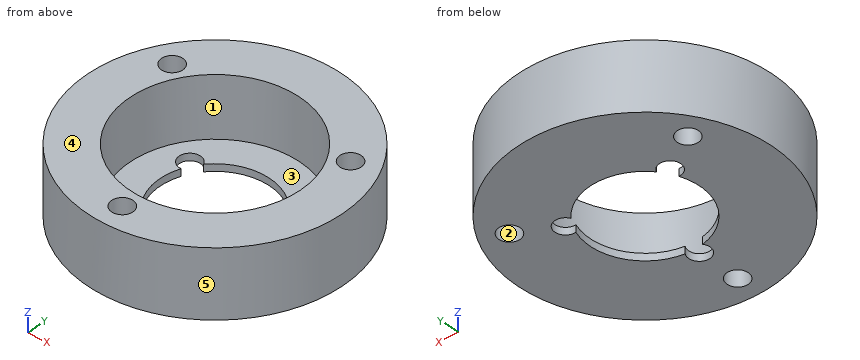
```python
from build123d import *

# Parameters (mm, degrees)
ESQUISSE1_W      = 50
ESQUISSE1_H      = 9.5
EXTRUSION1_DEPTH = 45
ESQUISSE2_R      = 1.5
EXTRUSION2_DEPTH = 45
ESQUISSE3_R      = 12
EXTRUSION3_DEPTH = 8.5
ESQUISSE4_R      = 36.120283588
ESQUISSE4_R_2    = 18
EXTRUSION4_DEPTH = 10.5


with BuildPart() as part:
    # Esquisse1 → Extrusion1 (new body)
    with BuildSketch(Plane(origin=(0, 0, 0), x_dir=(1, 0, 0), z_dir=(0, 1, 0))):
        with Locations((25, -4.75)):
            Rectangle(ESQUISSE1_W, ESQUISSE1_H)
    extrude(amount=EXTRUSION1_DEPTH)

    # Esquisse2 → Extrusion2 (cut)
    with BuildSketch(Plane.XY.offset(9.5)):
        with Locations((12.445, 29.74863263)):
            Circle(ESQUISSE2_R)
        with Locations((37.555, 29.74863263)):
            Circle(ESQUISSE2_R)
        with Locations((25, 8.002734741)):
            Circle(ESQUISSE2_R)
        with BuildLine():
            ThreePointArc((17.756055836, 25.254591249), (16.339745962, 27.5), (18.992481919, 27.396144045))
            ThreePointArc((18.992481919, 27.396144045), (25, 30.25), (31.007518081, 27.396144045))
            ThreePointArc((31.007518081, 27.396144045), (33.660254038, 27.5), (32.243944164, 25.254591249))
            ThreePointArc((32.243944164, 25.254591249), (31.711696879, 18.625), (26.236426083, 14.849264706))
            ThreePointArc((26.236426083, 14.849264706), (25, 12.5), (23.763573917, 14.849264706))
            ThreePointArc((23.763573917, 14.849264706), (18.288303121, 18.625), (17.756055836, 25.254591249))
        make_face()
    extrude(amount=-EXTRUSION2_DEPTH, mode=Mode.SUBTRACT)

    # Esquisse3 → Extrusion3 (cut)
    with BuildSketch(Plane.XY.offset(9.5)):
        with Locations((25, 22.5)):
            Circle(ESQUISSE3_R)
    extrude(amount=-EXTRUSION3_DEPTH, mode=Mode.SUBTRACT)

    # Esquisse4 → Extrusion4 (cut, through all)
    with BuildSketch(Plane.XY.offset(9.5)):
        with Locations((25, 22.5)):
            Circle(ESQUISSE4_R)
        with Locations((25, 22.5)):
            Circle(ESQUISSE4_R_2, mode=Mode.SUBTRACT)
    extrude(amount=-EXTRUSION4_DEPTH, mode=Mode.SUBTRACT)


solid = part.part
```
Input: part model. Units: mm. Frame: model coordinates. Face numbers are marked on the shaded views. A direction names the side the tool comes from. Coordinates: 2 decimals unless noted, no trailing zeros. Loops run counter-clockwise (first coordinate to the right, second up) from the corner with the lowest first, then second, coordinate; pieces in that order, holes last. Notation, with made-up numbers: (-20, 9.25) -> (-15, 9.25) arc R37 cw to (-15, 48.25) -> close; hole circle Ø8 at (-39.75, 51). An arc over 180 degrees is marked (long way). Use a Markdown table: item, result.
1) Cut plane C-C (z = 5.5). Return the cut outline in (x, y) (3 decimals).
Results found:
| item | result |
|---|---|
| outline | circle Ø36 at (25, 22.5); hole circle Ø3 at (12.445, 29.749); hole circle Ø24 at (25, 22.5); hole circle Ø3 at (25, 8.003); hole circle Ø3 at (37.555, 29.749) |
2) Material intervals for line 1 along Y through (x, z) = (25, 7.25); line 2 along X through (y, z) = (31, 8.75); line 3 along Z through (x, y) = (20, 32), sorted ascending. Write a range as from..to.
Results found:
| item | result |
|---|---|
| line 1 | y = 4.5..6.5, 9.5..10.5, 34.5..40.5 |
| line 2 | x = 9.13..11.62, 13.27..16.53, 33.47..36.73, 38.38..40.87 |
| line 3 | z = 0..1 |
3) Cut plane D-D (x = 35.5). Return the cut outline in (y, z), then the cut area to 3 significant figures.
Results found:
| item | result |
|---|---|
| outline | (7.88, 0) -> (37.12, 0) -> (37.12, 9.5) -> (28.31, 9.5) -> (28.31, 1) -> (16.69, 1) -> (16.69, 9.5) -> (7.88, 9.5) -> close |
| area | 179 mm2 |
4) Cut plane A-A (x = 25). Return the cut outline in (y, z).
Results found:
| item | result |
|---|---|
| outline | (4.5, 0) -> (6.5, 0) -> (6.5, 9.5) -> (4.5, 9.5) -> close; (9.5, 0) -> (12.5, 0) -> (12.5, 1) -> (10.5, 1) -> (10.5, 9.5) -> (9.5, 9.5) -> close; (30.25, 0) -> (40.5, 0) -> (40.5, 9.5) -> (34.5, 9.5) -> (34.5, 1) -> (30.25, 1) -> close |
5) Access query for the marked faces 1 and 2. Directions: +Z, -Z, +X, -X, +Y, -Y. A direction counts if a zero-diameter tool reaches every point of the face in a straight line with its end or side. Return the directions, or none.
Results found:
| item | result |
|---|---|
| face 1 | +Z |
| face 2 | +Z, -Z |
6) Cut plane B-B (y = 22.5). Return the cut outline in (x, z).
Results found:
| item | result |
|---|---|
| outline | (7, 0) -> (17.25, 0) -> (17.25, 1) -> (13, 1) -> (13, 9.5) -> (7, 9.5) -> close; (32.75, 0) -> (43, 0) -> (43, 9.5) -> (37, 9.5) -> (37, 1) -> (32.75, 1) -> close |
7) Pull-direction query (Y, two-part tool) for the marked faces 3, 4 and 5; classes: released by +Y, released by -Y, zero draft, split by the parting line, or undercut.
Results found:
| item | result |
|---|---|
| face 3 | undercut |
| face 4 | zero draft |
| face 5 | split by the parting line |
8) Contact query for flat-ended pins moving along their axis: pin 1 (10 mm diameter, centred on x = 24.5, y = 16, fed in from +Z); pin 2 (5 mm diameter, centred on y = 12.5, z = 7, fed in from -X); pin 3 (4 mm diameter, centred on x = 26, z = 4, fed in from -Y). Output: stop coordinate, or through.
Results found:
| item | result |
|---|---|
| pin 1 | stops at z = 1 |
| pin 2 | stops at x = 8.64 |
| pin 3 | stops at y = 4.5 |
